Check sheet for the modelled part. Datum: model origin and axes. Units: mm. A direction names the side the tool comes from. Round coordinates to 2 decimals unless told otherwise and drop trailing zeros. Order: outer loops, then holes, each group sorted by start corner. A loop starts at its lowest first (then second) coordinate and runs counter-clockwise, first axis right, second up. Notation, with made-up numbers: (68, 41.5) -> (83, 41.5) arc R7 cw to (83, 47.5) -> close; hole circle Ø8 at (-8.5, 72.5). An arc over 180 degrees is marked (long way). Use CSV: the item, a comma, the result in double quotes.
```python
from build123d import *

# Parameters (mm, degrees)
BOX572_W                     = 6
BOX572_H                     = 8
BOX572_DEPTH                 = 2
BOX572_PLACEMENT_ANGLE       = 45
BOX570_W                     = 6
BOX570_H                     = 8
BOX570_DEPTH                 = 2
BOX569_W                     = 6
BOX569_H                     = 8
BOX569_DEPTH                 = 2
BOX573_W                     = 6
BOX573_H                     = 8
BOX573_DEPTH                 = 2
BOX573_PLACEMENT_ANGLE       = 135
BOX574_W                     = 6
BOX574_H                     = 8
BOX574_DEPTH                 = 2
BOX571_W                     = 6
BOX571_H                     = 8
BOX571_DEPTH                 = 2
BOX571_PLACEMENT_ANGLE       = 225
BOX575_W                     = 6
BOX575_H                     = 8
BOX575_DEPTH                 = 2
BOX568_W                     = 6
BOX568_H                     = 8
BOX568_DEPTH                 = 2
BOX568_PLACEMENT_ANGLE       = 45
COMPOUND948_PLACEMENT_ANGLE  = 22.5
CYLINDER1361_R               = 1.5
CYLINDER1361_DEPTH           = 32
CYLINDER1361_PLACEMENT_ANGLE = 45
CYLINDER1364_R               = 1.5
CYLINDER1364_DEPTH           = 32
CYLINDER1362_R               = 1.5
CYLINDER1362_DEPTH           = 32
CYLINDER1362_PLACEMENT_ANGLE = 135
CYLINDER1360_R               = 1.5
CYLINDER1360_DEPTH           = 32
CYLINDER1358_R               = 1.5
CYLINDER1358_DEPTH           = 32
CYLINDER1358_PLACEMENT_ANGLE = 225
CYLINDER1363_R               = 1.5
CYLINDER1363_DEPTH           = 32
CYLINDER1357_R               = 1.5
CYLINDER1357_DEPTH           = 32
CYLINDER1357_PLACEMENT_ANGLE = 45
CYLINDER1359_R               = 1.5
CYLINDER1359_DEPTH           = 32
COMPOUND949_PLACEMENT_ANGLE  = 22.5
TUBE124_R                    = 50
TUBE124_R_2                  = 40
TUBE124_DEPTH                = 11
TUBE123_R                    = 46
TUBE123_R_2                  = 40
TUBE123_DEPTH                = 16


with BuildPart() as krychle572:
    # Box572 → Box572 (new body)
    with BuildSketch(Plane.XY):
        with Locations((3, 4)):
            Rectangle(BOX572_W, BOX572_H)
    extrude(amount=BOX572_DEPTH)


with BuildPart() as krychle572_1:
    # Box572 placement: moved
    add(krychle572.part.moved(Location((30.405592, -34.648232, 33))).rotate(Axis((30.405592, -34.648232, 33), (0, 0, 1)), BOX572_PLACEMENT_ANGLE))


with BuildPart() as krychle570:
    # Box570 → Box570 (new body)
    with BuildSketch(Plane(origin=(46, -3, 33), x_dir=(0, 1, 0), z_dir=(0, 0, 1))):
        with Locations((3, 4)):
            Rectangle(BOX570_W, BOX570_H)
    extrude(amount=BOX570_DEPTH)


with BuildPart() as krychle569:
    # Box569 → Box569 (new body)
    with BuildSketch(Plane(origin=(-3, -46, 33), x_dir=(1, 0, 0), z_dir=(0, 0, 1))):
        with Locations((3, 4)):
            Rectangle(BOX569_W, BOX569_H)
    extrude(amount=BOX569_DEPTH)


with BuildPart() as krychle573:
    # Box573 → Box573 (new body)
    with BuildSketch(Plane.XY):
        with Locations((3, 4)):
            Rectangle(BOX573_W, BOX573_H)
    extrude(amount=BOX573_DEPTH)


with BuildPart() as krychle573_1:
    # Box573 placement: moved
    add(krychle573.part.moved(Location((34.648232, 30.405592, 33))).rotate(Axis((34.648232, 30.405592, 33), (0, 0, 1)), BOX573_PLACEMENT_ANGLE))


with BuildPart() as krychle574:
    # Box574 → Box574 (new body)
    with BuildSketch(Plane(origin=(3, 46, 33), x_dir=(-1, 0, 0), z_dir=(0, 0, 1))):
        with Locations((3, 4)):
            Rectangle(BOX574_W, BOX574_H)
    extrude(amount=BOX574_DEPTH)


with BuildPart() as krychle571:
    # Box571 → Box571 (new body)
    with BuildSketch(Plane.XY):
        with Locations((3, 4)):
            Rectangle(BOX571_W, BOX571_H)
    extrude(amount=BOX571_DEPTH)


with BuildPart() as krychle571_1:
    # Box571 placement: moved
    add(krychle571.part.moved(Location((-30.405592, 34.648232, 33))).rotate(Axis((-30.405592, 34.648232, 33), (0, 0, 1)), BOX571_PLACEMENT_ANGLE))


with BuildPart() as krychle575:
    # Box575 → Box575 (new body)
    with BuildSketch(Plane(origin=(-46, 3, 33), x_dir=(0, -1, 0), z_dir=(0, 0, 1))):
        with Locations((3, 4)):
            Rectangle(BOX575_W, BOX575_H)
    extrude(amount=BOX575_DEPTH)


with BuildPart() as compound948:
    # Box568 → Box568 (new body)
    with BuildSketch(Plane.XY):
        with Locations((3, 4)):
            Rectangle(BOX568_W, BOX568_H)
    extrude(amount=BOX568_DEPTH)


with BuildPart() as compound948_1:
    # Box568 placement: moved
    add(compound948.part.moved(Location((-34.648232, -30.405592, 33))).rotate(Axis((-34.648232, -30.405592, 33), (0, 0, -1)), BOX568_PLACEMENT_ANGLE))

    # Compound948: union Krychle572, Krychle570, Krychle569, Krychle573, Krychle574, Krychle571, Krychle575
    add(krychle572_1.part)
    add(krychle570.part)
    add(krychle569.part)
    add(krychle573_1.part)
    add(krychle574.part)
    add(krychle571_1.part)
    add(krychle575.part)


with BuildPart() as compound948_2:
    # Compound948 placement: moved
    add(compound948_1.part.moved(Location((0, 0, 4.4))).rotate(Axis((0, 0, 4.4), (0, 0, 1)), COMPOUND948_PLACEMENT_ANGLE))


with BuildPart() as obj1:
    # Cylinder1361 → Cylinder1361 (new body)
    with BuildSketch(Plane.XY):
        Circle(CYLINDER1361_R)
    extrude(amount=CYLINDER1361_DEPTH)


with BuildPart() as obj1_1:
    # Cylinder1361 placement: moved
    add(obj1.part.moved(Location((29.698485, -29.698485, 33.5))).rotate(Axis((29.698485, -29.698485, 33.5), (0, 0, 1)), CYLINDER1361_PLACEMENT_ANGLE))


with BuildPart() as obj2:
    # Cylinder1364 → Cylinder1364 (new body)
    with BuildSketch(Plane(origin=(42, 0, 33.5), x_dir=(0, 1, 0), z_dir=(0, 0, 1))):
        Circle(CYLINDER1364_R)
    extrude(amount=CYLINDER1364_DEPTH)


with BuildPart() as obj3:
    # Cylinder1362 → Cylinder1362 (new body)
    with BuildSketch(Plane.XY):
        Circle(CYLINDER1362_R)
    extrude(amount=CYLINDER1362_DEPTH)


with BuildPart() as obj3_1:
    # Cylinder1362 placement: moved
    add(obj3.part.moved(Location((29.698485, 29.698485, 33.5))).rotate(Axis((29.698485, 29.698485, 33.5), (0, 0, 1)), CYLINDER1362_PLACEMENT_ANGLE))


with BuildPart() as obj4:
    # Cylinder1360 → Cylinder1360 (new body)
    with BuildSketch(Plane(origin=(0, 42, 33.5), x_dir=(-1, 0, 0), z_dir=(0, 0, 1))):
        Circle(CYLINDER1360_R)
    extrude(amount=CYLINDER1360_DEPTH)


with BuildPart() as obj5:
    # Cylinder1358 → Cylinder1358 (new body)
    with BuildSketch(Plane.XY):
        Circle(CYLINDER1358_R)
    extrude(amount=CYLINDER1358_DEPTH)


with BuildPart() as obj5_1:
    # Cylinder1358 placement: moved
    add(obj5.part.moved(Location((-29.698485, 29.698485, 33.5))).rotate(Axis((-29.698485, 29.698485, 33.5), (0, 0, 1)), CYLINDER1358_PLACEMENT_ANGLE))


with BuildPart() as obj6:
    # Cylinder1363 → Cylinder1363 (new body)
    with BuildSketch(Plane(origin=(-42, 0, 33.5), x_dir=(0, -1, 0), z_dir=(0, 0, 1))):
        Circle(CYLINDER1363_R)
    extrude(amount=CYLINDER1363_DEPTH)


with BuildPart() as obj7:
    # Cylinder1357 → Cylinder1357 (new body)
    with BuildSketch(Plane.XY):
        Circle(CYLINDER1357_R)
    extrude(amount=CYLINDER1357_DEPTH)


with BuildPart() as obj7_1:
    # Cylinder1357 placement: moved
    add(obj7.part.moved(Location((-29.698485, -29.698485, 33.5))).rotate(Axis((-29.698485, -29.698485, 33.5), (0, 0, -1)), CYLINDER1357_PLACEMENT_ANGLE))


with BuildPart() as compound949:
    # Cylinder1359 → Cylinder1359 (new body)
    with BuildSketch(Plane(origin=(0, -42, 33.5), x_dir=(1, 0, 0), z_dir=(0, 0, 1))):
        Circle(CYLINDER1359_R)
    extrude(amount=CYLINDER1359_DEPTH)

    # Compound949: union obj1, obj2, obj3, obj4, obj5, obj6, obj7
    add(obj1_1.part)
    add(obj2.part)
    add(obj3_1.part)
    add(obj4.part)
    add(obj5_1.part)
    add(obj6.part)
    add(obj7_1.part)


with BuildPart() as compound949_1:
    # Compound949 placement: moved
    add(compound949.part.rotate(Axis((0, 0, 0), (0, 0, 1)), COMPOUND949_PLACEMENT_ANGLE))


with BuildPart() as tube124:
    # Tube124 → Tube124 (new body)
    with BuildSketch(Plane.XY.offset(25.4)):
        Circle(TUBE124_R)
        Circle(TUBE124_R_2, mode=Mode.SUBTRACT)
    extrude(amount=TUBE124_DEPTH)


with BuildPart() as cut496:
    # Tube123 → Tube123 (new body)
    with BuildSketch(Plane.XY.offset(26)):
        Circle(TUBE123_R)
        Circle(TUBE123_R_2, mode=Mode.SUBTRACT)
    extrude(amount=TUBE123_DEPTH)

    # Cut493: cut Tube124
    add(tube124.part, mode=Mode.SUBTRACT)

    # Cut495: cut Compound949
    add(compound949_1.part, mode=Mode.SUBTRACT)

    # Cut496: cut Compound948
    add(compound948_2.part, mode=Mode.SUBTRACT)


with BuildPart() as cut496_1:
    # Cut496 placement: moved
    add(cut496.part.moved(Location((0, 0, 3))))


solid = cut496_1.part
```
Q1. Access from +Z, -Z, +X, -X, +Y, -Y to the whole of each face (thin tool, end or side, straight path). Record for faces 1 (the face through (-19.203, 38.52, 41.386)), 2 (the face through (38.52, 19.203, 41.386)), 3 (the face through (-41, 16, 42.4)), 4 (the face through (-38.52, 19.203, 41.386)).
Result sheet:
face 1,"+Y"
face 2,"+X"
face 3,"none"
face 4,"-X"
Q2. Scan lines: L1, parallel to X at y = -0.5, z = 42.15; L2, parallel to Y at x = 7, z = 43.9; L3, parallel to Y at x = 18, z = 44.4. Record each from-to range of solid material in increasing order.
Result sheet:
L1,"x = -46 to -40, 40 to 46"
L2,"y = -45.46 to -39.38, 39.38 to 45.46"
L3,"y = -42.33 to -35.72, 35.72 to 42.33"
Q3. Mould release check, pull along Z, two halves, no side actions. Record for faces 5 (the face through (-14.844, -37.943, 39.893)), 6 (the face through (38.52, -19.203, 41.386)): pulls with the +Z half, pulls with the -Z half, needs draft (parallel to the pull), parting line crosses it, or undercut.
Result sheet:
face 5,"needs draft"
face 6,"undercut"
Q4. Go/stop test with flat-tipped pins: pin 1 (10 mm diameter, centred on x = -24, y = 30.5, fed in from -Z); pin 2 (1.5 mm diameter, centred on y = 37, z = 41, fed in from +X); pin 3 (1 mm diameter, centred on y = -15.5, z = 44, fed in from +X); pin 4 (2 mm diameter, centred on y = -17, z = 44.5, fed in from -X). Record where each tip stops, or that it passes through.
Result sheet:
pin 1,"stops at z = 39.4"
pin 2,"stops at x = 28.32"
pin 3,"stops at x = 43.49"
pin 4,"stops at x = -43.13"
Q5. Sectioned sample at A-A, the plane x = 0. Enter the section's corners in (y, z).
Result sheet:
outline,"(-46, 39.4) -> (-40, 39.4) -> (-40, 45) -> (-46, 45) -> close; (40, 39.4) -> (46, 39.4) -> (46, 45) -> (40, 45) -> close"
Q6. Sectioned sample at C-C, the plane z = 41.25. State how many separate pieces and enclosed holes the cut face has, then the cut area to 3 significant figures.
Result sheet:
separate pieces,"8"
enclosed holes,"0"
area,"1,330 mm^2"
